Here's how the part is built. I have some questions about the finished solid (model axes, mm). A direction names the side the tool comes from. Round coordinates to 2 decimals unless told otherwise and drop trailing zeros. Loops run counter-clockwise (first coordinate to the right, second up) from the corner with the lowest first, then second, coordinate; pieces in that order, holes last. Notation, with made-up numbers: (60, 58.25) -> (76, 58.25) arc R25 ccw to (76, 72.25) -> close; hole circle Ø1 at (46, 55.5). An arc over 180 degrees is marked (long way). Use one line per item in the form item = value. Start each with the question number.
Item 1: For faces 4 (the face through (-55, 493, 133.75)), 5 (the face through (-42.5, 493, 166)), 6 (the face through (-191.45, 507, 190.76)), which set-ups out of +Z, -Z, +X, -X, +Y, -Y let a thin tool reach every point of the face, with its end or its side?
Item 2: If we section it at A-A (x = 0): Write out the boundary of the cut face in (y, z).
Item 3: I'm going to push flat-ended pins straight in: pin 1 Ø1 at (y, z) = (322.5, -11) entering from +X; pin 2 Ø3 at (x, z) = (-45.5, -13.5) entering from +Y. Where does each tip first touch, or does it pass through?
Item 4: If I drill on L1, parallel to Z at x = -133, y = 731; L2, parallel to X at y = 317.5, z = 134.5; L3, parallel to X at y = 664, z = -133, over which ranges is the centre line in solid material (lowest first)? Write a range as [from, to].
Item 5: Thinking about a two-plate mould opening in X: for faces 1 (the face through (193.69, 507, 191.23)), 2 (the face through (-190.979, 507, -191.445)), 3 (the face through (42.5, 493, 167)), which applies, released by +X, released by -X, zero draft, split by the parting line, or undercut?
Item 6: If we section it at C-C (y = 133.5): State how many separate pieces and enclosed holes the cut face has, then the cut area to 3 significant figures.
Item 7: If we section it at B-B (z = 143): Write out the boundary of the cut face in (x, y).
```python
from build123d import *

# Parameters (mm, degrees)
F1_DEPTH = 1000
F2_R     = 50
F2_R_2   = 52.5
F3_DEPTH = 2000
F4_R     = 30


with BuildPart() as f1:
    # F0 (on Front) → F1 (new body)
    with BuildSketch(Plane.XZ):
        with BuildLine():
            Line((-200, -133.75), (-200, -200))
            Line((-200, -200), (-42.5, -200))
            Line((-42.5, -200), (-42.5, -133.75))
            Line((-42.5, -133.75), (-67.5, -133.297282))
            Line((-67.5, -133.297282), (-67.5, -98.492385))
            Line((-67.5, -98.492385), (-30.746254, -62.88615))
            ThreePointArc((-30.746254, -62.88615), (-49.801599, -49.19147), (-63.260358, -29.96877))
            Line((-63.260358, -29.96877), (-100.854047, -67.608259))
            Line((-100.854047, -67.608259), (-133.75, -67.608259))
            Line((-133.75, -67.608259), (-133.75, -42.5))
            Line((-133.75, -42.5), (-200, -42.5))
            Line((-200, -42.5), (-200, -133.75))
        make_face()
        with BuildLine():
            ThreePointArc((-63.260358, -29.96877), (-49.801599, -49.19147), (-30.746254, -62.88615))
            ThreePointArc((-30.746254, -62.88615), (-1.031839, -69.992395), (28.879141, -63.765157))
            ThreePointArc((28.879141, -63.765157), (50.203622, -48.781106), (64.5687, -27.034847))
            ThreePointArc((64.5687, -27.034847), (68.628744, -13.787512), (70, 0))
            ThreePointArc((70, 0), (68.43998, 14.695888), (63.829453, 28.736751))
            ThreePointArc((63.829453, 28.736751), (49.94511, 49.045754), (29.891725, 63.296799))
            ThreePointArc((29.891725, 63.296799), (1.135837, 69.990784), (-27.822117, 64.233401))
            ThreePointArc((-27.822117, 64.233401), (-49.28701, 49.707048), (-63.994991, 28.366197))
            ThreePointArc((-63.994991, 28.366197), (-69.99445, -0.881465), (-63.260358, -29.96877))
        make_face()
        with BuildLine():
            ThreePointArc((64.5687, -27.034847), (50.203622, -48.781106), (28.879141, -63.765157))
            Line((28.879141, -63.765157), (67.5, -102.077139))
            Line((67.5, -102.077139), (67.5, -133.75))
            Line((67.5, -133.75), (42.5, -133.75))
            Line((42.5, -133.75), (42.5, -200))
            Line((42.5, -200), (202.712331, -200))
            Line((202.712331, -200), (202.712331, -42.5))
            Line((202.712331, -42.5), (136.462331, -42.5))
            Line((136.462331, -42.5), (136.462331, -67.608259))
            Line((136.462331, -67.608259), (105.641152, -67.608259))
            Line((105.641152, -67.608259), (64.5687, -27.034847))
        make_face()
        with BuildLine():
            Line((-103.335165, 67.391741), (-63.994991, 28.366197))
            ThreePointArc((-63.994991, 28.366197), (-49.28701, 49.707048), (-27.822117, 64.233401))
            Line((-27.822117, 64.233401), (-67.5, 103.429188))
            Line((-67.5, 103.429188), (-67.5, 133.75))
            Line((-67.5, 133.75), (-42.5, 133.75))
            Line((-42.5, 133.75), (-42.5, 199.783482))
            Line((-42.5, 199.783482), (-200, 199.783482))
            Line((-200, 199.783482), (-200, 42.5))
            Line((-200, 42.5), (-133.75, 42.5))
            Line((-133.75, 42.5), (-133.75, 67.391741))
            Line((-133.75, 67.391741), (-103.335165, 67.391741))
        make_face()
        with BuildLine():
            Line((67.5, 100.950892), (29.891725, 63.296799))
            ThreePointArc((29.891725, 63.296799), (49.94511, 49.045754), (63.829453, 28.736751))
            Line((63.829453, 28.736751), (103.730209, 67.391741))
            Line((103.730209, 67.391741), (136.462331, 67.391741))
            Line((136.462331, 67.391741), (136.462331, 42.5))
            Line((136.462331, 42.5), (202.712331, 41.300298))
            Line((202.712331, 41.300298), (202.712331, 199.783482))
            Line((202.712331, 199.783482), (42.5, 199.783482))
            Line((42.5, 199.783482), (42.5, 133.75))
            Line((42.5, 133.75), (67.5, 133.75))
            Line((67.5, 133.75), (67.5, 100.950892))
        make_face()
    extrude(amount=-F1_DEPTH)

    # F2 (on face) → F3 (cut)
    with BuildSketch(Plane.XZ):
        Circle(F2_R)
        with Locations((-133.75, 133.75)):
            Circle(F2_R_2)
        with Locations((133.75, 133.75)):
            Circle(F2_R_2)
        with Locations((133.75, -133.75)):
            Circle(F2_R_2)
        with Locations((-133.75, -133.75)):
            Circle(F2_R_2)
    extrude(amount=-F3_DEPTH, mode=Mode.SUBTRACT)

    # F4
    f4_edges = [f1.edges().sort_by_distance(p)[0] for p in [
        (202.712331, 500, 199.783482),
        (-200, 500, 199.783482),
        (202.712331, 500, -200),
        (-200, 500, -200),
    ]]
    fillet(f4_edges, radius=F4_R)


solid = f1.part
```
Values found:
q1.face_4 = +Y, -Y
q1.face_5 = +Z, +Y, -Y
q1.face_6 = +Z, -X, +Y, -Y
q2.outline = (0, -70) -> (1000, -70) -> (1000, -50) -> (0, -50) -> close; (0, 50) -> (1000, 50) -> (1000, 70) -> (0, 70) -> close
q3.pin_1 = 69.21
q3.pin_2 = through
q4.L1 = [-200, -186.24], [-81.26, -67.61], [67.39, 81.26], [186.24, 199.78]
q4.L2 = [-200, -186.24], [-81.26, -42.5], [42.5, 81.26], [186.24, 202.71]
q4.L3 = [-200, -186.24], [-81.26, -67.5], [67.5, 81.26], [186.24, 202.71]
q5.face_1 = released by +X
q5.face_2 = released by -X
q5.face_3 = undercut
q6.separate_pieces = 1
q6.enclosed_holes = 5
q6.area = 64,000 mm2
q7.outline = (-200, 0) -> (-185.43, 0) -> (-185.43, 1000) -> (-200, 1000) -> close; (-82.07, 0) -> (-42.5, 0) -> (-42.5, 1000) -> (-82.07, 1000) -> close; (42.5, 0) -> (82.07, 0) -> (82.07, 1000) -> (42.5, 1000) -> close; (185.43, 0) -> (202.71, 0) -> (202.71, 1000) -> (185.43, 1000) -> close
